Source: CAD feature listing. Evaluate the final solid. Frame: model axes, mm. A direction names the side the tool comes from. Coordinates: 2 decimals unless noted, no trailing zeros. Order: outer loops, then holes, each group sorted by start corner. A loop starts at its lowest first (then second) coordinate and runs counter-clockwise, first axis right, second up. Notation, with made-up numbers: (52, -3) - (60, -3) arc R25 ccw to (60, 29) - close; hole circle Ø5 at (70.25, 25). An arc over 180 degrees is marked (long way). One line per question, with ' | ' between items.
from build123d import *

# Parameters (mm, degrees)
F0_W     = 200
F0_H     = 300
F1_DEPTH = 250
F2_R     = 82.5
F3_DEPTH = 25
F5_DEPTH = 300.001
F6_R     = 25
F7_DEPTH = 100
F8_R     = 20


with BuildPart() as f1:
    # F0 (on Front) → F1 (new body)
    with BuildSketch(Plane.XZ):
        with Locations((100, 150)):
            Rectangle(F0_W, F0_H)
    extrude(amount=-F1_DEPTH)

    # F2 (on face) → F3 (join)
    with BuildSketch(Plane.XZ):
        with Locations((100, 200)):
            Circle(F2_R)
    extrude(amount=F3_DEPTH)

    # F4 (on face) → F5 (cut, through all)
    with BuildSketch(Plane.XY.offset(300)):
        Polygon((200, 250), (0, 250), (200, 100), align=None)
    extrude(amount=-F5_DEPTH, mode=Mode.SUBTRACT)

    # F6 (on face) → F7 (cut)
    with BuildSketch(Plane.XZ):
        with Locations((150, 50)):
            Circle(F6_R)
        with Locations((50, 50)):
            Circle(F6_R)
    extrude(amount=-F7_DEPTH, mode=Mode.SUBTRACT)

    # F8
    f8_edges = [f1.edges().sort_by_distance(p)[0] for p in [
        (25, 0, 50),
        (125, 0, 50),
        (17.5, -25, 200),
    ]]
    fillet(f8_edges, radius=F8_R)


solid = f1.part
(1) Material intervals for L1, parallel to X at y = 68, z = 60.5; L2, parallel to Z at x = 150, y = 56; L3, parallel to Z at x = 145, y = 97, sorted ascending. Write a range as from..to.
Taken from the geometry:
L1: x = 0..27.31, 72.69..127.31, 172.69..200 | L2: z = 0..25, 75..300 | L3: z = 0..25.51, 74.49..300
(2) Cut plane D-D (z = 200). Return the cut outline in (x, y), and give its area (3 significant figures).
Taken from the geometry:
outline: (0, 0) - (17.5, 0) - (17.5, -5) arc R20 ccw to (37.5, -25) - (162.5, -25) arc R20 ccw to (182.5, -5) - (182.5, 0) - (200, 0) - (200, 100) - (0, 250) - close | area: 39,000 mm²
(3) Pull-direction query (X, two-part tool) for faces 1 (the flat face through (200, 49, 148)), 2 (the flat face through (76, 0, 119)), 3 (the flat face through (150, 100, 50)); classes: pulls with the +X half, pulls with the -X half, needs draft (parallel to the pull), parting line crosses it, or undercut.
Taken from the geometry:
face 1: pulls with the +X half | face 2: needs draft | face 3: undercut
(4) Set-up query: faces 4 (the flat face through (0, 123, 148)), 5 (the cylindrical face through (144.58, 59.44, 25.594)). Return all of +Z, -Z, +X, -X, +Y, -Y with unobstructed straight access to the full face (end or side cutting, diameter ignored); none if empty.
Taken from the geometry:
face 4: +Z, -Z, -X, +Y, -Y | face 5: -Y
(5) Pin query (flat end, axial travel): P1, Ø8, axis at y = 209, z = 222, coming from the +X side; P2, Ø3, axis at x = 75.5, z = 31.5, coming from the -Y side; P3, Ø2, axis at x = 143.5, z = 260, coming from the -Y side. Return the tip coordinate at first contact, or that it passes through.
Taken from the geometry:
P1: stops at x = 60 | P2: stops at y = 4 | P3: stops at y = -21.95
(6) Cut plane C-C (x = 100). Return the cut outline in (y, z).
Taken from the geometry:
outline: (-25, 137.5) arc R20 ccw to (-5, 117.5) - (0, 117.5) - (0, 0) - (175, 0) - (175, 300) - (0, 300) - (0, 282.5) - (-5, 282.5) arc R20 ccw to (-25, 262.5) - close
(7) Cut plane A-A (z = 50). Return the cut outline in (x, y).
Taken from the geometry:
outline: (0, 0) - (5, 0) arc R20 ccw to (25, 20) - (25, 100) - (75, 100) - (75, 20) arc R20 ccw to (95, 0) - (105, 0) arc R20 ccw to (125, 20) - (125, 100) - (175, 100) - (175, 20) arc R20 ccw to (195, 0) - (200, 0) - (200, 100) - (0, 250) - close
(8) Cut plane B-B (y = 46). Return the cut outline in (x, z).
Taken from the geometry:
outline: (0, 0) - (200, 0) - (200, 300) - (0, 300) - close; hole circle Ø50 at (50, 50); hole circle Ø50 at (150, 50)
